Can you work these out from the model? Positions are in its coordinate system, mm. Face numbers are marked on the shaded views. Give positions to 0.01 mm unless a question says otherwise; leave off trailing zeros. Write each loop counter-clockwise with the first axis right and the second up, starting at its lowest first coordinate (ties: lowest second). Pieces come first, ordered by that corner, then holes.
from build123d import *

# Parameters (mm, degrees)
F0_R     = 10.16
F1_DEPTH = 25.4
F3_DEPTH = 152.4


with BuildPart() as f1:
    # F0 (on Front) → F1 (new body)
    with BuildSketch(Plane.XZ):
        with BuildLine():
            Line((0, 146.05), (0, 25.4))
            ThreePointArc((0, 25.4), (7.439488, 7.439488), (25.4, 0))
            Line((25.4, 0), (254, 0))
            ThreePointArc((254, 0), (271.960512, 7.439488), (279.4, 25.4))
            Line((279.4, 25.4), (279.4, 59.22473))
            ThreePointArc((279.4, 59.22473), (275.117971, 73.338244), (263.715646, 82.693139))
            Line((263.715646, 82.693139), (110.67542, 146.05))
            Line((110.67542, 146.05), (0, 146.05))
        make_face()
        with Locations((25.4, 38.1)):
            Circle(F0_R, mode=Mode.SUBTRACT)
        with Locations((63.5, 38.1)):
            Circle(F0_R, mode=Mode.SUBTRACT)
        with Locations((101.6, 38.1)):
            Circle(F0_R, mode=Mode.SUBTRACT)
        with Locations((139.7, 38.1)):
            Circle(F0_R, mode=Mode.SUBTRACT)
        with Locations((177.8, 38.1)):
            Circle(F0_R, mode=Mode.SUBTRACT)
        with Locations((215.9, 38.1)):
            Circle(F0_R, mode=Mode.SUBTRACT)
        with Locations((254, 38.1)):
            Circle(F0_R, mode=Mode.SUBTRACT)
    extrude(amount=F1_DEPTH)

    # F2 (on face) → F3 (cut)
    with BuildSketch(Plane(origin=(0, 0, 0), x_dir=(0, -1, 0), z_dir=(-1, 0, 0))):
        with BuildLine():
            Line((25.146, 146.05), (0.254, 146.05))
            ThreePointArc((0.254, 146.05), (12.7, 144.272), (25.146, 146.05))
        make_face()
    extrude(amount=-F3_DEPTH, mode=Mode.SUBTRACT)


solid = f1.part
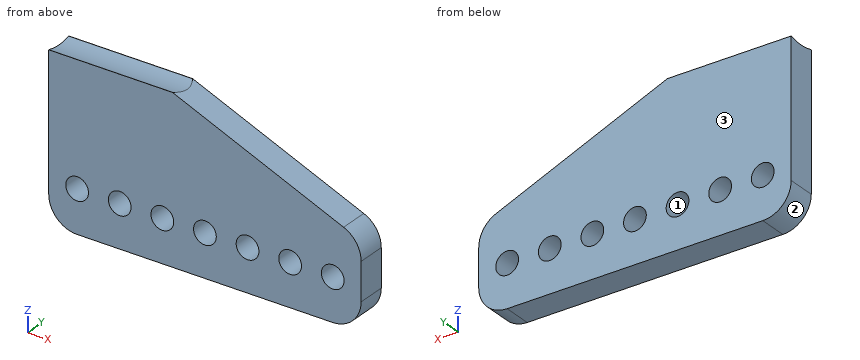
(1) Imagine slicing it at A-A, the plane x = 63.5. Write out the boundary of the cut face in (y, z), plus the area to 3 significant figures.
Returned:
outline: (-25.4, 0) - (0, 0) - (0, 27.94) - (-25.4, 27.94) - close; (-25.4, 48.26) - (0, 48.26) - (0, 146.05) - (-0.25, 146.05) arc R44.45 cw to (-25.15, 146.05) - (-25.4, 146.05) - close
area: 3,160 mm2
(2) Imagine slicing it at D-D, the plane x = 177.8. Write out the boundary of the cut face in (y, z).
Returned:
outline: (-25.4, 0) - (0, 0) - (0, 27.94) - (-25.4, 27.94) - close; (-25.4, 48.26) - (0, 48.26) - (0, 118.26) - (-25.4, 118.26) - close
(3) If we mould it in two halves opening along X, with no side actions, what happens to the marked faces 1, 2 and 3? For each: +X half, -X half, draft (parallel to the pull), parting line (faces both ways), or undercut.
Returned:
face 1: undercut
face 2: -X half
face 3: draft
(4) Imagine slicing it at B-B, the plane z = 38.1. Give the number of separate pieces and of enclosed holes in the cut face, plus the area to 3 significant figures.
Returned:
separate pieces: 8
enclosed holes: 0
area: 3,480 mm2
(5) If I drill on L1, parallel to Z at x = 52, y = -11.75; L2, parallel to Z at x = 132, y = -3.5; L3, parallel to Z at x = 59.5, y = -7, over which ranges is the centre line in solid material (lowest first)?
Returned:
L1: z = 0 to 144.28
L2: z = 0 to 31.47, 44.73 to 137.22
L3: z = 0 to 28.76, 47.44 to 144.64
(6) Imagine slicing it at C-C, the plane y = -5.25. Write out the boundary of the cut face in (x, z).
Returned:
outline: (0, 25.4) arc R25.4 ccw to (25.4, 0) - (254, 0) arc R25.4 ccw to (279.4, 25.4) - (279.4, 59.22) arc R25.4 ccw to (263.72, 82.69) - (113.45, 144.9) - (0, 144.9) - close; hole circle Ø20.32 at (25.4, 38.1); hole circle Ø20.32 at (63.5, 38.1); hole circle Ø20.32 at (101.6, 38.1); hole circle Ø20.32 at (139.7, 38.1); hole circle Ø20.32 at (177.8, 38.1); hole circle Ø20.32 at (215.9, 38.1); hole circle Ø20.32 at (254, 38.1)
(7) Will this pin go through, and if not, where does the flat tip stop? P1, Ø5, axis at x = 44, y = -10.5, coming from the +Z side.
Returned:
P1: stops at z = 144.52
